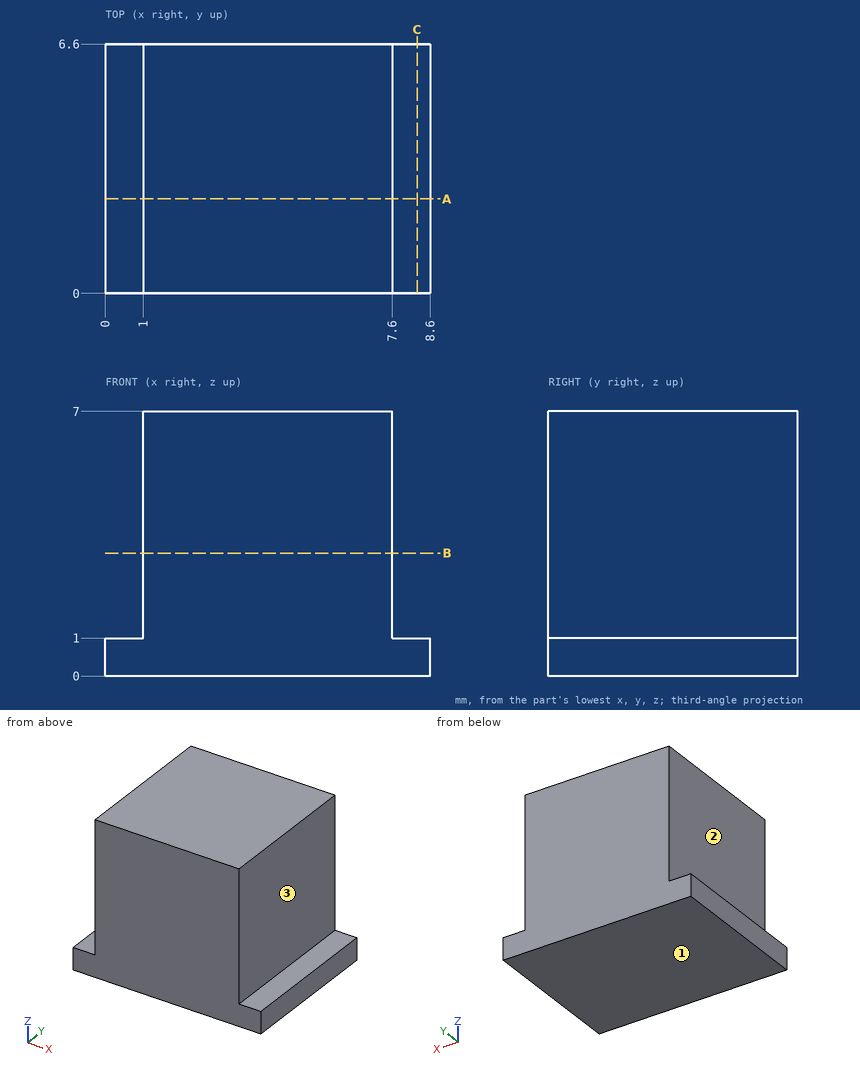
Geometry check sheet. Reference: drawing and pictorial views, mm from the part's lowest x, y, z. A direction names the side the tool comes from. Round coordinates to 2 decimals unless told otherwise and drop trailing zeros. Order: outer loops, then holes, each group sorted by start corner. A loop starts at its lowest first (then second) coordinate and runs counter-clockwise, first axis right, second up. Notation, with made-up numbers: M 83.5,27 L 97.5,27 A29 ccw 97.5,58 Z; hole C 13,22 d5. An arc over 180 degrees is marked long. Write item = value, one per line.
Q1. Scan line: line 1 (X direction, y = 1.25, z = 3.5). Record every from-to range of solid material in increasing order.
Answer block:
line_1 = 1 to 7.6
Q2. Depth check by flat-ended pin: pin 1 Ø0.5 at (x, y) = (0.5, 3) entering from +Z; pin 2 Ø1 at (y, z) = (1.5, 2) entering from +X; pin 3 Ø1.5 at (y, z) = (3.5, 3.5) entering from -X. Enter the tip coordinate at first touch or a pass-through.
Answer block:
pin_1 = 1
pin_2 = 7.6
pin_3 = 1
Q3. Section check C-C (x = 8.25). Enter the section's corners in (y, z), plus the area to 3 significant figures.
Answer block:
outline = M 0,0 L 6.6,0 L 6.6,1 L 0,1 Z
area = 6.60 mm^2
Q4. Set-up check for the marked faces 1, 2 and 3: record each of +Z, -Z, +X, -X, +Y, -Y from which the full face is reachable in a straight line by a thin tool's end or side.
Answer block:
face_1 = -Z, +X, -X, +Y, -Y
face_2 = +Z, -X, +Y, -Y
face_3 = +Z, +X, +Y, -Y
Q5. Section check A-A (y = 2.5). Enter the section's corners in (x, z), plus the area to 3 significant figures.
Answer block:
outline = M 0,0 L 8.6,0 L 8.6,1 L 7.6,1 L 7.6,7 L 1,7 L 1,1 L 0,1 Z
area = 48.2 mm^2
Q6. Section check B-B (z = 3.25). Enter the section's corners in (x, y), plus the area to 3 significant figures.
Answer block:
outline = M 1,0 L 7.6,0 L 7.6,6.6 L 1,6.6 Z
area = 43.6 mm^2
